Verification items for this drawing (mm, ordinates from the low corner). A direction names the side the tool comes from. Give positions to 0.01 mm unless a question says otherwise; leave off trailing zeros. Order: outer loops, then holes, each group sorted by start corner. A loop starts at its lowest first (then second) coordinate and runs counter-clockwise, first axis right, second up. Notation, with made-up numbers: (-30, 18) -> (9, 18) arc R21 ccw to (9, 35) -> close; hole circle Ø7 at (32.5, 0.25). An arc over 180 degrees is marked (long way). One line per question, with ' | ' between items.
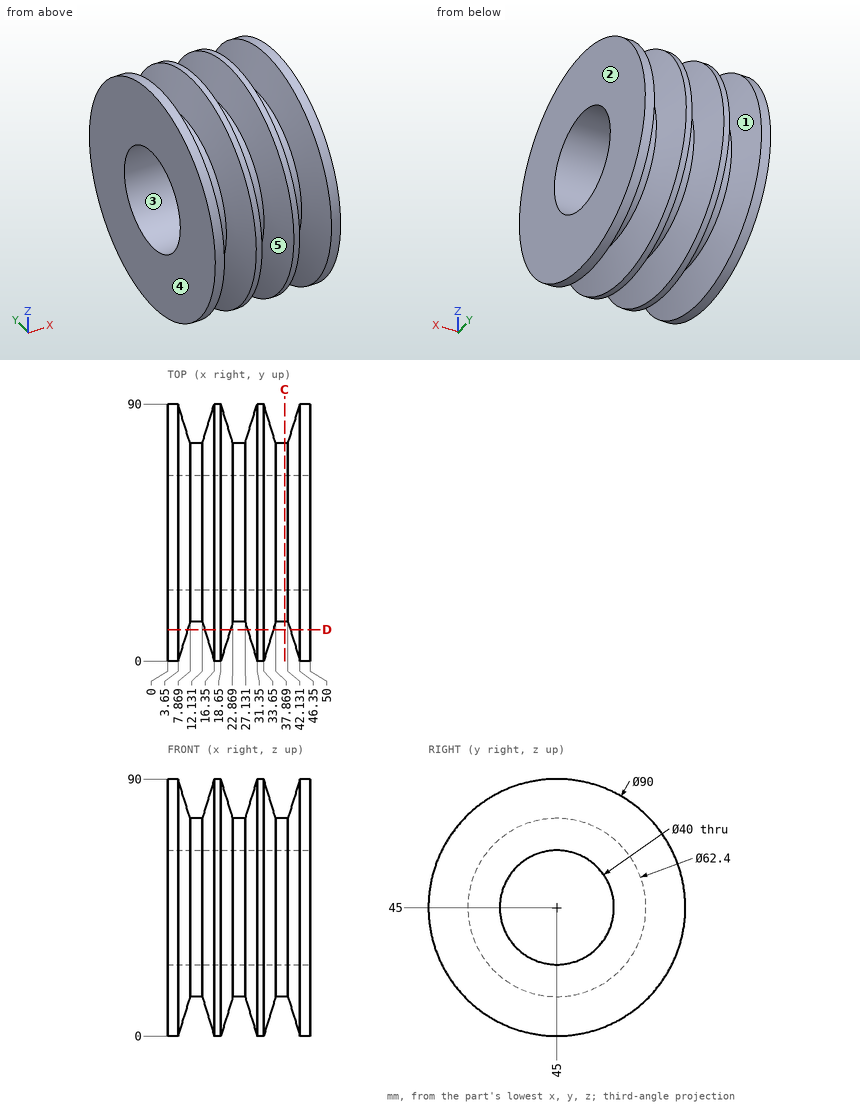
Q1. Section check C-C (x = 41). Enter the section's corners in (y, z).
Result sheet:
outline: circle Ø62.4 at (45, 45); hole circle Ø40 at (45, 45)
Q2. Thickness scan on line 1 (X direction, y = 74, z = 61); line 2 (X direction, y = 15, z = 63.5); line 3 (Y direction, x = 39, z = 45). Record the ranges inside material, lowest first.
Result sheet:
line 1: x = 0 to 7.28, 12.72 to 22.28, 27.72 to 37.28, 42.72 to 50 | line 2: x = 0 to 6.63, 13.37 to 21.63, 28.37 to 36.63, 43.37 to 50 | line 3: y = 13.8 to 25, 65 to 76.2
Q3. Mould release check, pull along Y, two halves, no side actions. Record for the marked faces 3, 4 and 5: pulls with the +Y half, pulls with the -Y half, needs draft (parallel to the pull), parting line crosses it, or undercut.
Result sheet:
face 3: undercut | face 4: needs draft | face 5: parting line crosses it
Q4. Section check D-D (y = 11). Count the separate pieces of the cut face and the enclosed holes in it, and give its area (3 significant figures).
Result sheet:
separate pieces: 4 | enclosed holes: 0 | area: 1,470 mm2
Q5. Depth check by flat-ended pin: pin 1 Ø12 at (x, z) = (39, 77) entering from +Y; pin 2 Ø6 at (x, z) = (32, 15) entering from -Y; pin 3 Ø3 at (y, z) = (28.5, 53) entering from +X; pin 4 Ø4 at (x, z) = (33.5, 17) entering from -Y. Enter the tip coordinate at first touch or a pass-through.
Result sheet:
pin 1: stops at y = 79.17 | pin 2: stops at y = 9 | pin 3: passes through | pin 4: stops at y = 8.27
Q6. Access from +Z, -Z, +X, -X, +Y, -Y to the whole of each face (thin tool, end or side, straight path). Record for the marked faces 1 and 2.
Result sheet:
face 1: none | face 2: +Z, -Z, +X, +Y, -Y
